Input: part model. Units: mm. Frame: model coordinates. A direction names the side the tool comes from. Round coordinates to 2 decimals unless told otherwise and drop trailing zeros. Loops run counter-clockwise (first coordinate to the right, second up) from the corner with the lowest first, then second, coordinate; pieces in that order, holes last. Notation, with made-up numbers: (-27.75, 71) -> (22.25, 71) arc R24 cw to (22.25, 102) -> close; hole circle Ø6 at (-26.5, 54). An arc over 180 degrees is marked (long way). Answer as a JSON object with one key per item and string values.
Autodesk Inventor part; units mm, degrees
ref_plane "YZ Plane" through (0, 0, 0) normal (1, 0, 0) x (0, 1, 0)
ref_plane "XZ Plane" through (0, 0, 0) normal (0, 1, 0) x (-1, 0, 0)
ref_plane "XY Plane" through (0, 0, 0) normal (0, 0, 1) x (1, 0, 0)
sketch "Sketch1" plane through (0, 0, 0) normal (0, 1, 0) x (-1, 0, 0)
  line L0 (35.0198, 16.1328) -> (-28.4802, 16.1328)
  line L1 (-28.4802, 16.1328) -> (-28.4802, -15.6172)
  line L2 (-28.4802, -15.6172) -> (35.0198, -15.6172)
  line L3 (35.0198, -15.6172) -> (35.0198, 16.1328)
  point P0 (0, 0)
  dimension "d0" = 63.5
  dimension "d1" = 31.75
extrude "Extrusion1" add sketch "Sketch1" along normal blind 38.1
sketch "Sketch2" plane through (0, 38.1, 0) normal (0, 1, 0) x (1, 0, 0)
  line L0 (28.4802, -16.1328) -> (28.4802, 15.6172)
  line L1 (15.7802, 15.6172) -> (15.7802, 9.2672)
  line L2 (28.4802, 9.2672) -> (28.4802, 15.6172)
  line L3 (15.7802, 15.6172) -> (-22.3198, 15.6172)
  line L4 (-22.3198, 15.6172) -> (-22.3198, -16.1328)
  line L5 (-22.3198, -16.1328) -> (15.7802, -16.1328)
  line L6 (15.7802, -16.1328) -> (15.7802, 15.6172)
  point P0 (0, 0)
  dimension "d4" = 12.7
  dimension "d5" = 6.35
  dimension "d6" = 38.1
  dimension "d7" = 31.75
extrude "Extrusion2" cut sketch "Sketch2" against normal blind 25.4
sketch "Sketch3" plane through (28.4802, 0, 16.1328) normal (1, 0, 0) x (0, 0, -1)
  line L0 (0, 12.7) -> (0, 38.1)
  circle A0 centre (0, 38.1) radius 25.4
  point P0 (16.1328, 0)
  dimension "d10" = 50.8
extrude "Extrusion3" cut sketch "Sketch3" against normal blind 76.2
sketch "Sketch4" plane through (0, 12.7, 0) normal (0, 1, 0) x (1, 0, 0)
  line L0 (28.4802, 15.6172) -> (-35.0198, 15.6172)
  line L1 (15.8725, 15.6172) -> (3.1725, 15.6172)
  line L2 (15.8725, 2.9172) -> (15.8725, 15.6172)
  line L3 (3.1725, 2.9172) -> (-9.5275, 2.9172)
  line L4 (-9.5275, 2.9172) -> (-9.5275, -9.7828)
  line L5 (-9.5275, -9.7828) -> (3.1725, -9.7828)
  line L6 (3.1725, -9.7828) -> (3.1725, 2.9172)
  point P0 (0, 0)
  dimension "d13" = 12.7
  dimension "d14" = 12.7
  dimension "d15" = 12.7
  dimension "d16" = 12.7
extrude "Extrusion4" cut sketch "Sketch4" against normal blind 25.4
1) Section B-B, the plane x = 0. Output: boundary loops of the cut face in (y, z), plus the area to 3 significant figures.
Output:
{"outline": "(0, -15.62) -> (12.7, -15.62) -> (12.7, -2.92) -> (0, -2.92) -> close; (0, 9.78) -> (12.7, 9.78) -> (12.7, 16.13) -> (0, 16.13) -> close", "area": "242 mm^2"}
2) Ray query, probe 1 along X at (y, z) = (6, 5); probe 2 along X at (y, z) = (13, -6); probe 3 along Y at (x, z) = (12, 12.5). Return the intervals inside material, ascending.
Output:
{"probe 1": "x = -35.02 to -9.53, 3.17 to 28.48", "probe 2": "x = -35.02 to -22.32, 15.78 to 28.48", "probe 3": "y = 0 to 12.7"}
3) Contact query for flat-ended pins moving along their axis: P1, Ø7.5, axis at y = 20.5, z = -0.5, coming from the +X side; P2, Ø12.5, axis at y = 27.5, z = 7, coming from the -X side. Output: stop coordinate, or through.
Output:
{"P1": "stops at x = 28.48", "P2": "passes through"}
4) Section A-A, the plane y = 32. Output: boundary loops of the cut face in (x, z), plus the area to 3 significant figures.
Output:
{"outline": "(-35.02, -15.62) -> (-22.32, -15.62) -> (-22.32, -8.52) -> (-35.02, -8.52) -> close; (15.78, -15.62) -> (28.48, -15.62) -> (28.48, -8.52) -> (15.78, -8.52) -> close", "area": "180 mm^2"}
5) Section C-C, the plane z = 2. Output: boundary loops of the cut face in (x, y), plus the area to 3 significant figures.
Output:
{"outline": "(-35.02, 0) -> (-9.53, 0) -> (-9.53, 12.7) -> (-22.32, 12.7) -> (-22.32, 16.99) -> (-35.02, 16.99) -> close; (3.17, 0) -> (28.48, 0) -> (28.48, 16.99) -> (15.78, 16.99) -> (15.78, 12.7) -> (3.17, 12.7) -> close", "area": "754 mm^2"}
6) Reachability of faces 4 (the face through (-3, 6, 9.783)), 5 (the face through (15.78, 23, -7)), 6 (the face through (-35.02, 15, -3)) from +Z, -Z, +X, -X, +Y, -Y: full face, straight path, thin tool, end or side. Return the list, or none.
Output:
{"face 4": "+Y, -Y", "face 5": "+Z, -Z, +Y", "face 6": "+Z, -Z, -X, +Y, -Y"}
7) Section D-D, the plane z = -11. Output: boundary loops of the cut face in (x, y), plus the area to 3 significant figures.
Output:
{"outline": "(-35.02, 0) -> (28.48, 0) -> (28.48, 38.1) -> (15.78, 38.1) -> (15.78, 12.7) -> (-22.32, 12.7) -> (-22.32, 38.1) -> (-35.02, 38.1) -> close", "area": "1,450 mm^2"}
8) Draft query along Z for faces 1 (the face through (28.48, 15, -3)), 2 (the face through (22.219, 19.943, -1.629)), 3 (the face through (3.172, 6, 4)). Return one class per face: +Z half, -Z half, draft (parallel to the pull), parting line (faces both ways), or undercut.
Output:
{"face 1": "draft", "face 2": "+Z half", "face 3": "undercut"}
